Could you check a few things on this model? Use its own coordinates, in mm. Face numbers are marked on the shaded views. A direction names the side the tool comes from. Round coordinates to 2 decimals unless told otherwise and drop trailing zeros. Write each loop counter-clockwise with the first axis right and the second up, starting at its lowest first coordinate (ties: lowest second). Pieces come first, ordered by that corner, then holes. Notation, with made-up numbers: (70.5, 85) -> (111.5, 85) arc R27 ccw to (111.5, 106) -> close; hole circle Ø4 at (27, -38.75). An arc over 180 degrees is marked (long way). Answer as CSV lines item,"result". Start each with the question number.
Q1. Will these pins go through, and if not, where does the flat tip stop? pin 1 Ø5 at (y, z) = (4.5, 3) entering from -X; pin 2 Ø1.5 at (y, z) = (19.5, 6) entering from +X; pin 3 Ø1.5 at (x, z) = (7.5, -7) entering from +Y; pin 4 Ø4 at (x, z) = (14.5, 7.5) entering from +Y.
Q2. Imagine slicing it at C-C on z = -2.5. Please give me the cut outline in (x, y).
Q3. If I drill on line 1 (Z direction, x = 1.75, y = 21.5); line 2 (X direction, y = 3.25, z = -6); line 3 (Z direction, x = 7.5, y = 18), over which ranges is the centre line in solid material (lowest first)? Write a range as [from, to].
Q4. Imagine slicing it at A-A on x = 14.5. Please give me the cut outline in (y, z), and give its area (4 significant figures).
Q5. For the marked faces 1 and 2, which set-ups out of +Z, -Z, +X, -X, +Y, -Y let a thin tool reach every point of the face, with its end or its side?
Q6. Imagine slicing it at B-B on y = 11.5. Please give me the cut outline in (x, z).
Q7. If we mould it in two halves opening along X, with no side actions, what happens to the marked faces 3, 4, 5 and 6? For each: pulls with the +X half, pulls with the -X half, needs draft (parallel to the pull), parting line crosses it, or undercut.
Q8. Imagine slicing it at D-D on z = -7.5. Please give me the cut outline in (x, y).
from build123d import *

# Parameters (mm, degrees)
BOSS_EXTRUDE1_DEPTH = 16.5
CUT_EXTRUDE1_REACH  = 42.525
SKETCH2_R           = 1.75
CUT_EXTRUDE2_REACH  = 42.525
SKETCH6_R           = 1.75
BOSS_EXTRUDE2_DEPTH = 5.5
CHAMFER1_SIZE       = 1.5


with BuildPart() as part:
    # Sketch1 → Boss-Extrude1 (new, symmetric)
    with BuildSketch(Plane.XY):
        Polygon((0, 0), (0, 29), (6, 29), (6, 6), (29, 6), (29, 0), align=None)
    extrude(amount=BOSS_EXTRUDE1_DEPTH, both=True)

    # Sketch2 → Cut-Extrude1 (cut, up to next)
    with BuildSketch(Plane(origin=(6, 0, 0), x_dir=(0, 0, -1), z_dir=(1, 0, 0)), mode=Mode.PRIVATE) as cut_extrude1_sk1:
        with Locations(Location((7.5, 21.5, 0), (0, 0, 90))):
            Circle(SKETCH2_R)
    cut_extrude1_tool1 = extrude(cut_extrude1_sk1.sketch, amount=-CUT_EXTRUDE1_REACH, mode=Mode.PRIVATE) & part.part
    # Sketch2 → Cut-Extrude1 (cut, up to next)
    with BuildSketch(Plane(origin=(6, 0, 0), x_dir=(0, 0, -1), z_dir=(1, 0, 0)), mode=Mode.PRIVATE) as cut_extrude1_sk2:
        with Locations(Location((7.5, 11.5, 0), (0, 0, 90))):
            Circle(SKETCH2_R)
    cut_extrude1_tool2 = extrude(cut_extrude1_sk2.sketch, amount=-CUT_EXTRUDE1_REACH, mode=Mode.PRIVATE) & part.part
    # Sketch2 → Cut-Extrude1 (cut, up to next)
    with BuildSketch(Plane(origin=(6, 0, 0), x_dir=(0, 0, -1), z_dir=(1, 0, 0)), mode=Mode.PRIVATE) as cut_extrude1_sk3:
        with Locations(Location((-7.5, 11.5, 0), (0, 0, 90))):
            Circle(SKETCH2_R)
    cut_extrude1_tool3 = extrude(cut_extrude1_sk3.sketch, amount=-CUT_EXTRUDE1_REACH, mode=Mode.PRIVATE) & part.part
    # Sketch2 → Cut-Extrude1 (cut, up to next)
    with BuildSketch(Plane(origin=(6, 0, 0), x_dir=(0, 0, -1), z_dir=(1, 0, 0)), mode=Mode.PRIVATE) as cut_extrude1_sk4:
        with Locations(Location((-7.5, 21.5, 0), (0, 0, 90))):
            Circle(SKETCH2_R)
    cut_extrude1_tool4 = extrude(cut_extrude1_sk4.sketch, amount=-CUT_EXTRUDE1_REACH, mode=Mode.PRIVATE) & part.part
    add(cut_extrude1_tool1.solids().sort_by_distance((6, 21.5, -7.5))[0], mode=Mode.SUBTRACT)
    add(cut_extrude1_tool2.solids().sort_by_distance((6, 11.5, -7.5))[0], mode=Mode.SUBTRACT)
    add(cut_extrude1_tool3.solids().sort_by_distance((6, 11.5, 7.5))[0], mode=Mode.SUBTRACT)
    add(cut_extrude1_tool4.solids().sort_by_distance((6, 21.5, 7.5))[0], mode=Mode.SUBTRACT)

    # Sketch6 → Cut-Extrude2 (cut, up to next)
    with BuildSketch(Plane(origin=(0, 6, 0), x_dir=(1, 0, 0), z_dir=(0, 1, 0)), mode=Mode.PRIVATE) as cut_extrude2_sk1:
        with Locations(Location((14.5, -7.5, 0), (0, 0, 180))):
            Circle(SKETCH6_R)
    cut_extrude2_tool1 = extrude(cut_extrude2_sk1.sketch, amount=-CUT_EXTRUDE2_REACH, mode=Mode.PRIVATE) & part.part
    # Sketch6 → Cut-Extrude2 (cut, up to next)
    with BuildSketch(Plane(origin=(0, 6, 0), x_dir=(1, 0, 0), z_dir=(0, 1, 0)), mode=Mode.PRIVATE) as cut_extrude2_sk2:
        with Locations(Location((14.5, 7.5, 0), (0, 0, 180))):
            Circle(SKETCH6_R)
    cut_extrude2_tool2 = extrude(cut_extrude2_sk2.sketch, amount=-CUT_EXTRUDE2_REACH, mode=Mode.PRIVATE) & part.part
    # Sketch6 → Cut-Extrude2 (cut, up to next)
    with BuildSketch(Plane(origin=(0, 6, 0), x_dir=(1, 0, 0), z_dir=(0, 1, 0)), mode=Mode.PRIVATE) as cut_extrude2_sk3:
        with Locations(Location((24.5, 7.5, 0), (0, 0, 180))):
            Circle(SKETCH6_R)
    cut_extrude2_tool3 = extrude(cut_extrude2_sk3.sketch, amount=-CUT_EXTRUDE2_REACH, mode=Mode.PRIVATE) & part.part
    # Sketch6 → Cut-Extrude2 (cut, up to next)
    with BuildSketch(Plane(origin=(0, 6, 0), x_dir=(1, 0, 0), z_dir=(0, 1, 0)), mode=Mode.PRIVATE) as cut_extrude2_sk4:
        with Locations(Location((24.5, -7.5, 0), (0, 0, 180))):
            Circle(SKETCH6_R)
    cut_extrude2_tool4 = extrude(cut_extrude2_sk4.sketch, amount=-CUT_EXTRUDE2_REACH, mode=Mode.PRIVATE) & part.part
    add(cut_extrude2_tool1.solids().sort_by_distance((14.5, 6, 7.5))[0], mode=Mode.SUBTRACT)
    add(cut_extrude2_tool2.solids().sort_by_distance((14.5, 6, -7.5))[0], mode=Mode.SUBTRACT)
    add(cut_extrude2_tool3.solids().sort_by_distance((24.5, 6, -7.5))[0], mode=Mode.SUBTRACT)
    add(cut_extrude2_tool4.solids().sort_by_distance((24.5, 6, 7.5))[0], mode=Mode.SUBTRACT)

    # Sketch3 → Boss-Extrude2 (add)
    with BuildSketch(Plane.XY.offset(16.5)):
        Polygon((6, 26), (26, 6), (6, 6), align=None)
    boss_extrude2 = extrude(amount=-BOSS_EXTRUDE2_DEPTH)

    # Mirror1: Boss-Extrude2 across plane
    add(boss_extrude2.mirror(Plane.XY))

    # Chamfer1
    chamfer1_edges = [part.edges().sort_by_distance(p)[0] for p in [
        (6, 6, 0),
    ]]
    chamfer(chamfer1_edges, length=CHAMFER1_SIZE)


solid = part.part
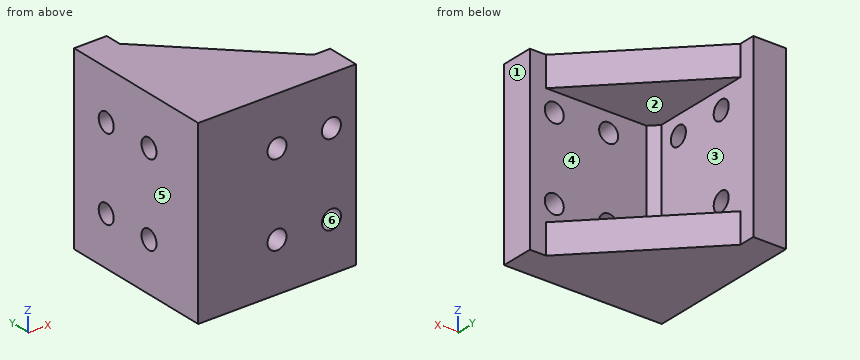
Checks:
1,pin 1,"x = 0"
1,pin 2,"x = 6"
1,pin 3,"y = 6.75"
1,pin 4,"y = 6"
2,outline,"(0, 0) -> (29, 0) -> (29, 6) -> (7.5, 6) -> (6, 7.5) -> (6, 29) -> (0, 29) -> close"
3,line 1,"[-16.5, -9.25], [-5.75, 5.75], [9.25, 16.5]"
3,line 2,"[0, 13.6], [15.4, 23.6], [25.4, 29]"
3,line 3,"[-16.5, -11], [11, 16.5]"
4,outline,"(0, -16.5) -> (17.5, -16.5) -> (17.5, -11) -> (6, -11) -> (6, -9.25) -> (0, -9.25) -> close; (0, -5.75) -> (6, -5.75) -> (6, 5.75) -> (0, 5.75) -> close; (0, 9.25) -> (6, 9.25) -> (6, 11) -> (17.5, 11) -> (17.5, 16.5) -> (0, 16.5) -> close"
4,area,"282.5 mm^2"
5,face 1,"+Z, -Z, +X, +Y, -Y"
5,face 2,"+X, +Y"
6,outline,"(0, -16.5) -> (20.5, -16.5) -> (20.5, -11) -> (6, -11) -> (6, -9.25) -> (0, -9.25) -> close; (0, -5.75) -> (6, -5.75) -> (6, 5.75) -> (0, 5.75) -> close; (0, 9.25) -> (6, 9.25) -> (6, 11) -> (20.5, 11) -> (20.5, 16.5) -> (0, 16.5) -> close"
7,face 3,"pulls with the +X half"
7,face 4,"needs draft"
7,face 5,"pulls with the -X half"
7,face 6,"undercut"
8,outline,"(0, 0) -> (12.75, 0) -> (12.75, 6) -> (7.5, 6) -> (6, 7.5) -> (6, 9.75) -> (0, 9.75) -> close; (0, 13.25) -> (6, 13.25) -> (6, 19.75) -> (0, 19.75) -> close; (0, 23.25) -> (6, 23.25) -> (6, 29) -> (0, 29) -> close; (16.25, 0) -> (22.75, 0) -> (22.75, 6) -> (16.25, 6) -> close; (26.25, 0) -> (29, 0) -> (29, 6) -> (26.25, 6) -> close"
